```python
from build123d import *

# Parameters (mm, degrees)
F1_DEPTH      = 4.7498
F2_R          = 0.889
F3_DEPTH      = 0.7874
F3_DEPTH_BACK = 25.4


with BuildPart() as f1:
    # F0 (on Right) → F1 (new body)
    with BuildSketch(Plane.YZ):
        Polygon((22.091185, 4.76885), (35.71647, 0), (73.82103, 0), (87.446315, 4.76885), (109.5375, 4.76885), (109.5375, 5.55625), (87.3125, 5.55625), (74.196499, 0.96565), (73.687214, 0.7874), (73.147637, 0.7874), (35.850286, 0.7874), (22.225, 5.55625), (0, 5.55625), (0, 4.76885), align=None)
    extrude(amount=F1_DEPTH)

    # F2 (on face) → F3 (cut, two sides)
    with BuildSketch(Plane.XY.offset(5.55625)) as f3_sk:
        with Locations((2.3749, 2.286)):
            Circle(F2_R)
        with Locations((2.3749, 107.2515)):
            Circle(F2_R)
        with Locations((2.3749, 90.9955)):
            Circle(F2_R)
        with Locations((2.3749, 18.542)):
            Circle(F2_R)
    extrude(amount=-F3_DEPTH, mode=Mode.SUBTRACT)
    extrude(f3_sk.sketch, amount=-F3_DEPTH_BACK, mode=Mode.SUBTRACT)


solid = f1.part
```
Input: part model. Units: mm. Frame: model coordinates. A direction names the side the tool comes from. Round coordinates to 2 decimals unless told otherwise and drop trailing zeros. Loops run counter-clockwise (first coordinate to the right, second up) from the corner with the lowest first, then second, coordinate; pieces in that order, holes last. Notation, with made-up numbers: (-33, 12) - (-19, 12) arc R16 cw to (-19, 41) - close; hole circle Ø1 at (17, -39). An arc over 180 degrees is marked (long way). One line per item, written item: value. Start each with the question number.
(1) Draft query along X for faces 1 (the cylindrical face through (2.182, 106.384, 5.168)), 2 (the flat face through (2.342, 28.808, 2.418)), 3 (the flat face through (4.75, 54.5, 0.5)). Return one class per face: +X half, -X half, draft (parallel to the pull), parting line (faces both ways), or undercut.
(2) Ray query, line 1 (X direction, y = 91, z = 5.15); line 2 (Z direction, x = 3.6, y = 97); line 3 (Z direction, x = 0.5, y = 62). Return the intervals inside material, ascending. Write a range as [from, to].
(3) Contact query for flat-ended pins moving along their axis: P1, Ø2, axis at x = 2.37, y = 18.54, coming from the -Z side; P2, Ø1.5, axis at x = 3, y = 60.5, coming from the +Z side. Output: stop coordinate, or through.
(4) Section C-C, the plane y = 81.5. Return loops of the section in (x, z), plus the area to 3 significant figures.
(5) Section B-B, the plane y = 13.5. Return loops of the section in (x, z).
(6) Section A-A, the plane z = 2.9. Return loops of the section in (x, y).
(7) Access query for faces 4 (the flat face through (2, 98, 4.769)), 5 (the flat face through (0, 54.5, 0.5)), 6 (the flat face through (2, 11, 4.769)), 7 (the flat face through (2, 99, 5.556)), 8 (the flat face through (2.34, 29.13, 3.14)). Directions: +Z, -Z, +X, -X, +Y, -Y. A direction counts if a zero-diameter tool reaches every point of the face in a straight line with its end or side. Return the directions, or none.
Results below:
1. face 1: undercut
1. face 2: draft
1. face 3: +X half
2. line 1: [0, 1.49], [3.26, 4.75]
2. line 2: [4.77, 5.56]
2. line 3: [0, 0.79]
3. P1: z = 4.77
3. P2: z = 0.79
4. outline: (0, 2.69) - (4.75, 2.69) - (4.75, 3.52) - (0, 3.52) - close
4. area: 3.96 mm^2
5. outline: (0, 4.77) - (4.75, 4.77) - (4.75, 5.56) - (0, 5.56) - close
6. outline: (0, 27.43) - (4.75, 27.43) - (4.75, 29.81) - (0, 29.81) - close; (0, 79.72) - (4.75, 79.72) - (4.75, 82.11) - (0, 82.11) - close
7. face 4: -Z, +X, -X, +Y
7. face 5: +Z, -Z, -X, +Y, -Y
7. face 6: -Z, +X, -X, -Y
7. face 7: +Z, +X, -X, +Y, -Y
7. face 8: +Z, +X, -X
